For this review, take the finished solid that the model builds, in its own axes (mm). A direction names the side the tool comes from. Coordinates: 2 decimals unless noted, no trailing zeros. Order: outer loops, then holes, each group sorted by start corner. A loop starts at its lowest first (then second) coordinate and runs counter-clockwise, first axis right, second up. Notation, with made-up numbers: (47, -33) -> (61, -33) arc R24 ccw to (61, -22) -> close; hole circle Ø8 at (13.5, 45.5). An arc over 180 degrees is marked (long way). Answer as a JSON object with one key per item and string values. Group by question number.
1) For pin 1 (1.5 mm diameter, centred on x = -3.5, z = 1.5, fed in from -Y); pin 2 (4 mm diameter, centred on x = -5, z = 3, fed in from +Y); pin 3 (0.9 mm diameter, centred on x = -5, y = 0, fed in from +Z), all flat-tipped, find the tip position at first contact; note any pin that passes through.
2) Draft analysis for pull direction X (two halves, no side actions). For faces 1 (the flat face through (-1, 0, 4)), 2 (the cylindrical face through (0.923, -1.774, 4.984)), 3 (the flat face through (1.3, 0, 8.25)), state which applies: +X half, -X half, draft (parallel to the pull), parting line (faces both ways), or undercut.
3) Add section B-B, the plane x = 0. Write out the cut boundary in (y, z).
4) Add section C-C, the plane z = 1.5. Write out the cut boundary in (x, y), then the cut area to 3 significant figures.
5) Add section A-A, the plane y = 0. Write out the cut boundary in (x, z), then the cut area to 3 significant figures.
6) Wall thickness on L1, parallel to X at y = 0.1, z = 1.5; L2, parallel to Z at x = -4.5, y = -0.5; L3, parallel to Y at x = 3, z = 3.25: over which ranges is each line inside the solid? List them lowest first.
7) Add section D-D, the plane x = 4. Write out the cut boundary in (y, z).
8) Machinability: for faces 4 (the flat face through (5, 1.5, 2)), 5 (the flat face through (5, -1.5, 2)), 6 (the flat face through (-5, 1.5, 2)), 7 (the flat face through (1, 0, 4)), which of the approach directions +Z, -Z, +X, -X, +Y, -Y give a long, thin tool a straight path to every point of the face, cutting with its end or side? Answer none if there is none.
from build123d import *

# Parameters (mm, degrees)
BOX001_W       = 2
BOX001_H       = 2
BOX001_DEPTH   = 10
BOX_W          = 16
BOX_H          = 3
BOX_DEPTH      = 5
CYLINDER_R     = 2
CYLINDER_DEPTH = 8.25


with BuildPart() as cube001:
    # Box001 → Box001 (new body)
    with BuildSketch(Plane(origin=(-1, -1, 0), x_dir=(1, 0, 0), z_dir=(0, 0, 1))):
        with Locations((1, 1)):
            Rectangle(BOX001_W, BOX001_H)
    extrude(amount=BOX001_DEPTH)


with BuildPart() as cube:
    # Box → Box (new body)
    with BuildSketch(Plane(origin=(-8, -1.5, 0), x_dir=(1, 0, 0), z_dir=(0, 0, 1))):
        with Locations((8, 1.5)):
            Rectangle(BOX_W, BOX_H)
    extrude(amount=BOX_DEPTH)


with BuildPart() as cut:
    # Cylinder → Cylinder (new body)
    with BuildSketch(Plane.XY):
        Circle(CYLINDER_R)
    extrude(amount=CYLINDER_DEPTH)

    # Fusion: union Cube
    add(cube.part)

    # Cut: cut Cube001
    add(cube001.part, mode=Mode.SUBTRACT)


solid = cut.part
Output values:
{
 "1": {"pin 1": "stops at y = -1.5", "pin 2": "stops at y = 1.5", "pin 3": "stops at z = 5"},
 "2": {"face 1": "undercut", "face 2": "parting line", "face 3": "draft"},
 "3": {"outline": "(-2, 0) -> (-1, 0) -> (-1, 8.25) -> (-2, 8.25) -> close; (1, 0) -> (2, 0) -> (2, 8.25) -> (1, 8.25) -> close"},
 "4": {"outline": "(-8, -1.5) -> (-1.32, -1.5) arc R2 ccw to (1.32, -1.5) -> (8, -1.5) -> (8, 1.5) -> (1.32, 1.5) arc R2 ccw to (-1.32, 1.5) -> (-8, 1.5) -> close; hole (-1, -1) -> (1, -1) -> (1, 1) -> (-1, 1) -> close", "area": "45.8 mm²"},
 "5": {"outline": "(-8, 0) -> (-1, 0) -> (-1, 8.25) -> (-2, 8.25) -> (-2, 5) -> (-8, 5) -> close; (1, 0) -> (8, 0) -> (8, 5) -> (2, 5) -> (2, 8.25) -> (1, 8.25) -> close", "area": "76.5 mm²"},
 "6": {"L1": "x = -8 to -1, 1 to 8", "L2": "z = 0 to 5", "L3": "y = -1.5 to 1.5"},
 "7": {"outline": "(-1.5, 0) -> (1.5, 0) -> (1.5, 5) -> (-1.5, 5) -> close"},
 "8": {"face 4": "+Z, -Z, +X, +Y", "face 5": "+Z, -Z, +X, -Y", "face 6": "+Z, -Z, -X, +Y", "face 7": "+Z, -Z"}
}
